Input: part model. Units: mm. Frame: model coordinates. Face numbers are marked on the shaded views. Give positions to 0.01 mm unless a question says otherwise; leave off trailing zeros. Loops run counter-clockwise (first coordinate to the right, second up) from the corner with the lowest first, then second, coordinate; pieces in that order, holes last. Notation, with made-up numbers: (-13, 77.25) -> (44, 77.25) arc R33 cw to (44, 115.25) -> close; hole circle Ø9 at (44, -32). An arc over 180 degrees is marked (long way). Answer as a JSON object with one key per item and string values.
```python
from build123d import *

# Parameters (mm, degrees)
SKETCH1_R           = 1.5
BOSS_EXTRUDE1_DEPTH = 3
BOSS_EXTRUDE2_DEPTH = 94


with BuildPart() as part:
    # Sketch1 → Boss-Extrude1 (new body)
    with BuildSketch(Plane(origin=(0, 0, 0), x_dir=(1, 0, 0), z_dir=(0, 1, 0))):
        Polygon((-51.61867002, -8.75119844), (-51.61867002, 3.502641742), (-66.587954735, 3.502641742), (-66.587954735, -4.206262026), align=None)
        with Locations((-54.587954735, 0.793737974)):
            Circle(SKETCH1_R, mode=Mode.SUBTRACT)
        with Locations((-60.587954735, 0.793737974)):
            Circle(SKETCH1_R, mode=Mode.SUBTRACT)
    boss_extrude1 = extrude(amount=BOSS_EXTRUDE1_DEPTH)

    # Sketch2 → Boss-Extrude2 (add)
    with BuildSketch(Plane(origin=(0, 3, 0), x_dir=(1, 0, 0), z_dir=(0, 1, 0))):
        Polygon((-64.087954735, 3.502641742), (-66.587954735, 3.502641742), (-66.587954735, -4.206262026), (-63.361180244, -5.185967146), (-61.932848842, -5.619633518), (-51.61867002, -8.75119844), (-51.61867002, -6.138508769), (-61.92070968, -3.010629509), (-64.087954735, -2.35261604), align=None)
    extrude(amount=BOSS_EXTRUDE2_DEPTH)

    # Mirror1: Boss-Extrude1 across plane
    add(boss_extrude1.mirror(Plane(origin=(0, 50, 0), x_dir=(0, 0, 1), z_dir=(0, -1, 0))))


solid = part.part
```
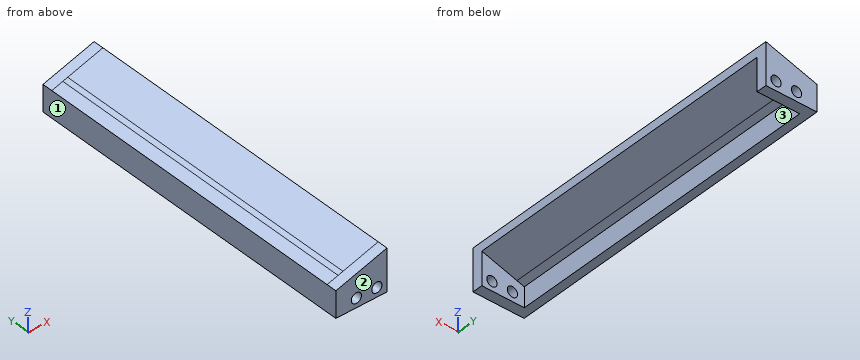
Q1. Draft query along Y for the marked faces 1, 2 and 3. Return one class per face: +Y half, -Y half, draft (parallel to the pull), parting line (faces both ways), or undercut.
Evaluation:
{"face 1": "draft", "face 2": "-Y half", "face 3": "undercut"}
Q2. Section C-C, the plane x = -58.25. Return the cut outline in (y, z).
Evaluation:
{"outline": "(0, -3.5) -> (3, -3.5) -> (3, 4.13) -> (97, 4.13) -> (97, -3.5) -> (100, -3.5) -> (100, 6.74) -> (0, 6.74) -> close"}
Q3. Pin query (flat end, axial travel): pin 1 (4 mm diameter, centred on x = -54, z = -0.5, fed in from +Y); pin 2 (1 mm diameter, centred on x = -61, y = 17, fed in from +Z); pin 3 (4 mm diameter, centred on x = -59, y = 62.5, fed in from -Z); pin 4 (3 mm diameter, centred on y = 42, z = -0.5, fed in from +X). Return the tip coordinate at first contact, or that it passes through.
Evaluation:
{"pin 1": "stops at y = 100", "pin 2": "stops at z = 6.05", "pin 3": "stops at z = 3.29", "pin 4": "stops at x = -64.09"}
Q4. Section A-A, the plane y = 64.5. Return the cut outline in (x, z), then the cut area to 3 significant figures.
Evaluation:
{"outline": "(-66.59, -3.5) -> (-64.09, -3.5) -> (-64.09, 2.35) -> (-51.62, 6.14) -> (-51.62, 8.75) -> (-66.59, 4.21) -> close", "area": "52.8 mm2"}
Q5. Ray query, line 1 along Y through (x, z) = (-60.5, 1.5); line 2 along X through (y, z) = (83, 1.5); line 3 along Z through (x, y) = (-54.75, 55). Return the intervals inside material, ascending.
Evaluation:
{"line 1": "y = 0 to 3, 97 to 100", "line 2": "x = -66.59 to -64.09", "line 3": "z = 5.19 to 7.8"}
Q6. Section D-D, the plane x = -65. Return the cut outline in (y, z), then the cut area to 3 significant figures.
Evaluation:
{"outline": "(0, -3.5) -> (100, -3.5) -> (100, 4.69) -> (0, 4.69) -> close", "area": "819 mm2"}
Q7. Section B-B, the plane x = -54. Return the cut outline in (y, z).
Evaluation:
{"outline": "(0, -3.5) -> (3, -3.5) -> (3, -2.17) -> (0, -2.17) -> close; (0, 0.59) -> (3, 0.59) -> (3, 5.42) -> (97, 5.42) -> (97, 0.59) -> (100, 0.59) -> (100, 8.03) -> (0, 8.03) -> close; (97, -3.5) -> (100, -3.5) -> (100, -2.17) -> (97, -2.17) -> close"}
